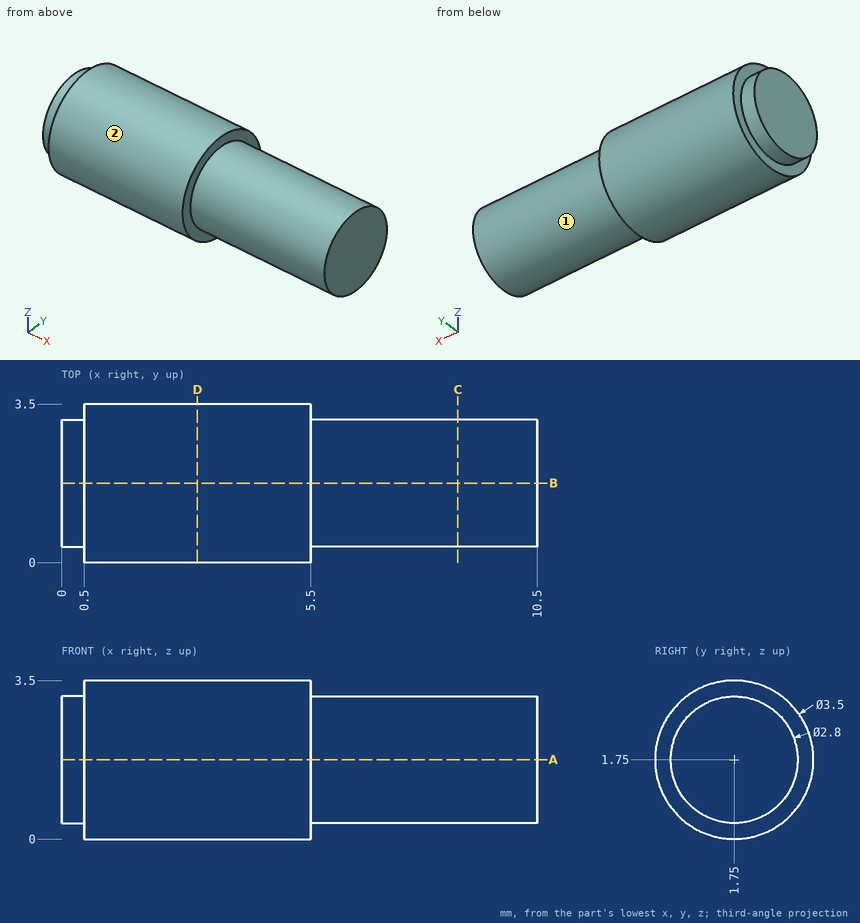
Geometry check sheet. Reference: drawing and pictorial views, mm from the part's lowest x, y, z. A direction names the side the tool comes from. Round coordinates to 2 decimals unless told otherwise and drop trailing zeros. Loops run counter-clockwise (first coordinate to the right, second up) from the corner with the lowest first, then second, coordinate; pieces in that order, holes last. Notation, with made-up numbers: (34, 30.5) - (85, 30.5) arc R34 ccw to (85, 68.5) - close; hole circle Ø11 at (12, 3.25). An arc over 180 degrees is marked (long way). Use a Markdown table: item, result.
Q1. Access from +Z, -Z, +X, -X, +Y, -Y to the whole of each face (thin tool, end or side, straight path). Record for the marked faces 1 and 2.
Solutions:
| item | result |
|---|---|
| face 1 | +X |
| face 2 | +X, -X |
Q2. Cross-section at D-D on x = 3. Record the cut outline in (y, z).
Solutions:
| item | result |
|---|---|
| outline | circle Ø3.5 at (1.75, 1.75) |
Q3. Material ranges on line 1 (X direction, y = 0.95, z = 3); line 2 (Y direction, x = 4.5, z = 1.85); line 3 (Z direction, x = 5.75, y = 0.8), recorded low to high.
Solutions:
| item | result |
|---|---|
| line 1 | x = 0.5 to 5.5 |
| line 2 | y = 0 to 3.5 |
| line 3 | z = 0.72 to 2.78 |
Q4. Cross-section at A-A on z = 1.75. Record the cut outline in (x, y).
Solutions:
| item | result |
|---|---|
| outline | (0, 0.35) - (0.5, 0.35) - (0.5, 0) - (5.5, 0) - (5.5, 0.35) - (10.5, 0.35) - (10.5, 3.15) - (5.5, 3.15) - (5.5, 3.5) - (0.5, 3.5) - (0.5, 3.15) - (0, 3.15) - close |
Q5. Go/stop test with flat-tipped pins: P1, Ø1, axis at x = 7, y = 1, coming from the -Z side; P2, Ø2, axis at x = 9, y = 0.5, coming from the +Z side. Record where each tip stops, or that it passes through.
Solutions:
| item | result |
|---|---|
| P1 | stops at z = 0.37 |
| P2 | stops at z = 3.13 |
Q6. Cross-section at C-C on x = 8.75. Record the cut outline in (y, z).
Solutions:
| item | result |
|---|---|
| outline | circle Ø2.8 at (1.75, 1.75) |
